Read the model definition and answer for the solid it produces. Units are mm, in the model's axes. Give positions to 0.01 mm unless a question says otherwise; leave off trailing zeros. Order: outer loops, then holes, each group sorted by start corner. A loop starts at its lowest first (then second) coordinate and runs counter-clockwise, first axis right, second up. Notation, with made-up numbers: M 20.25,27 L 71.25,27 A28 ccw 71.25,65 Z; hole C 76,43 d3. An arc over 180 degrees is marked long. Write item = value, one per line. Start each with the question number.
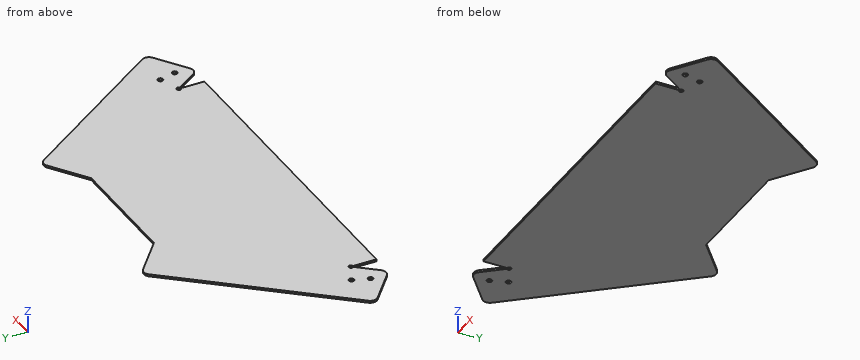
from build123d import *

# Parameters (mm, degrees)
F0_R     = 1.89865
F1_DEPTH = 1.5875
F2_R     = 5.08
F4_DEPTH = 1.5875


with BuildPart() as f1:
    # F0 (on Top) → F1 (new body)
    with BuildSketch(Plane.XY):
        Polygon((-33.3375, 56.7449798869), (-119.0625, -44.8550201131), (-119.0625, -63.9050201131), (125.4125, -63.9050201131), (125.4125, -44.8550201131), (55.5625, 56.7449798869), (46.0375, 56.7449798869), (17.4625, 56.7449798869), (0, 56.7449798869), align=None)
        Polygon((-135.4422218559, -64.2680237942), (-119.0625, -44.8550201131), (-33.3375, 56.7449798869), (-62.4570055217, 81.3145626708), (-164.5617273776, -39.6984410103), align=None)
        with Locations((-138.1131343099, -49.5519186622)):
            Circle(F0_R, mode=Mode.SUBTRACT)
        with Locations((-133.7370015814, -37.6296931006)):
            Circle(F0_R, mode=Mode.SUBTRACT)
        Polygon((55.5625, 56.7449798869), (125.4125, -44.8550201131), (139.7551548144, -65.8180411948), (171.1511521264, -44.2332930428), (86.9113565218, 78.2973187457), align=None)
        with Locations((143.8612788229, -51.4362030224)):
            Circle(F0_R, mode=Mode.SUBTRACT)
        with Locations((140.6796238031, -39.1412011381)):
            Circle(F0_R, mode=Mode.SUBTRACT)
    extrude(amount=F1_DEPTH)

    # F2
    f2_edges = [f1.edges().sort_by_distance(p)[0] for p in [
        (-164.561727, -39.698441, 0.79375),
        (-135.442222, -64.268024, 0.79375),
        (139.755155, -65.818041, 0.79375),
        (171.151152, -44.233293, 0.79375),
        (86.911357, 78.297319, 0.79375),
        (-62.457006, 81.314563, 0.79375),
    ]]
    fillet(f2_edges, radius=F2_R)

    # F3 (on face) → F4 (cut, through all)
    with BuildSketch(Plane.XY.offset(1.5875)):
        with BuildLine():
            ThreePointArc((127, -44.8550201131), (124.2899679849, -43.7324880979), (125.4125, -46.4425201131))
            Line((125.4125, -46.4425201131), (125.4125, -44.8550201131))
            Line((125.4125, -44.8550201131), (126.3089159259, -46.1652089307))
            ThreePointArc((126.3089159259, -46.1652089307), (126.816639689, -45.5956603657), (127, -44.8550201131))
        make_face()
        with BuildLine():
            ThreePointArc((-119.0625, -46.4425201131), (-117.9399679849, -45.9775521282), (-117.475, -44.8550201131))
            ThreePointArc((-117.475, -44.8550201131), (-119.7314472035, -43.4153444937), (-120.086232616, -46.0683328431))
            Line((-120.086232616, -46.0683328431), (-119.0625, -44.8550201131))
            Line((-119.0625, -44.8550201131), (-119.0625, -46.4425201131))
        make_face()
    extrude(amount=-F4_DEPTH, mode=Mode.SUBTRACT)


solid = f1.part
1) Find section B-B on z = 0.5. Determine the outline of the cut face in (x, y) (1 decimal).
2) Each of these flat-tipped pins is pushed along its axis until it touches: P1, Ø2.5, axis at x = 143.86, y = -51.44, coming from the -Z side; P2, Ø0.8, axis at x = -4.5, z = 1, coming from the +Y side (3 decimals); P3, Ø0.8, axis at y = -54.5, z = 0.5, coming from the -X side. Where does it stop, or does it pass through?
3) Find the intervals of material crossed by probe 1 along X at (y, z) = (-51, 1); probe 2 along X at (y, z) = (-53.5, 1.2); probe 3 along Y at (x, z) = (86, 1.4), in increasing order. Write a range as [from, to].
4) Find section A-A on y = 61. Determine the outline of the cut face in (x, z), plus the area to 3 significant figures.
5) Find section C-C on x = 12. Determine the outline of the cut face in (y, z), plus the area to 3 significant figures.
6) Find section D-D on y = 20. Determine the outline of the cut face in (x, z).
Numbers:
q1.outline = M -161.3,-35.8 A5.1 ccw -160.7,-43 L -139.3,-61 A5.1 ccw -132.2,-60.4 L -120.1,-46.1 A1.6 cw long -119.1,-46.4 L -119.1,-63.9 L 125.4,-63.9 L 125.4,-46.4 A1.6 cw long 126.3,-46.2 L 136.9,-61.6 A5.1 ccw 144,-62.9 L 167,-47.1 A5.1 ccw 168.3,-40 L 89.8,74.1 A5.1 ccw 82.7,75.4 L 55.6,56.7 L -33.3,56.7 L -58.6,78 A5.1 ccw -65.7,77.4 Z; hole C -138.1,-49.6 d3.8; hole C -133.7,-37.6 d3.8; hole C 140.7,-39.1 d3.8; hole C 143.9,-51.4 d3.8
q2.P1 = through
q2.P2 = 56.745
q2.P3 = -147.49
q3.probe_1 = [-151.17, -139.34], [-136.89, -124.25], [-119.06, 125.41], [129.62, 142.01], [145.71, 161.31]
q3.probe_2 = [-148.2, -126.36], [-119.06, 125.41], [131.33, 157.67]
q3.probe_3 = [-63.91, 76.3]
q4.outline = M -79.6,0 L -38.38,0 L -38.38,1.59 L -79.6,1.59 Z; M 61.75,0 L 98.8,0 L 98.8,1.59 L 61.75,1.59 Z
q4.area = 124 mm2
q5.outline = M -63.91,0 L 56.74,0 L 56.74,1.59 L -63.91,1.59 Z
q5.area = 192 mm2
q6.outline = M -114.19,0 L 126.99,0 L 126.99,1.59 L -114.19,1.59 Z
